Autodesk Inventor part; units mm, degrees
ref_plane "YZ Plane" through (0, 0, 0) normal (1, 0, 0) x (0, 1, 0)
ref_plane "XZ Plane" through (0, 0, 0) normal (0, 1, 0) x (-1, 0, 0)
ref_plane "XY Plane" through (0, 0, 0) normal (0, 0, 1) x (1, 0, 0)
sketch "스케치1" plane through (0, 0, 0) normal (0, 1, 0) x (-1, 0, 0)
  line L0 (0, 0) -> (-48, 0)
  line L1 (-48, 0) -> (-48, -6)
  line L2 (-48, -6) -> (0, -6)
  line L3 (0, -6) -> (0, 0)
  dimension "d0" = 48
  dimension "d1" = 6
extrude "돌출1" add sketch "스케치1" along normal blind 2
fillet "모깎기1" radius 1 7 edges at (0, 1, -6) (0, 1, 0) (0, 2, -3) (24, 2, -6) (48, 2, -3) (24, 2, 0) (48, 1, -6)
fillet "모깎기2" radius 1 2 edges at (47.7071, 1.7071, -0.2929) (48, 0.5, 0)
properties part number "gojung"
Can you work these out from the model? Positions are in its coordinate system, mm. Give positions to 0.01 mm unless a question says otherwise; leave off trailing zeros. Order: outer loops, then holes, each group sorted by start corner. A loop starts at its lowest first (then second) coordinate and runs counter-clockwise, first axis right, second up. Notation, with made-up numbers: M 84,5.5 L 127,5.5 A13 ccw 127,29.5 Z; hole C 87,53.25 d3. An arc over 180 degrees is marked long. One line per item, written item: value.
1) I want a section at A-A, the plane x = 33. List the corners of the cut face in (y, z) for me.
Answer sheet:
outline: M 0,-6 L 1,-6 A1 ccw 2,-5 L 2,-1 A1 ccw 1,0 L 0,0 Z
2) I want a section at B-B, the plane y = 1.6. List the corners of the cut face in (x, z) for me, plus the area to 3 significant figures.
Answer sheet:
outline: M 0.2,-5 A0.8 ccw 1,-5.8 L 47,-5.8 A0.8 ccw 47.8,-5 L 47.8,-1 A0.8 ccw 47,-0.2 L 1,-0.2 A0.8 ccw 0.2,-1 Z
area: 266 mm^2
3) I want a section at C-C, the plane z = -5.4. List the corners of the cut face in (x, y) for me, plus the area to 3 significant figures.
Answer sheet:
outline: M 0.08,0 L 47.92,0 L 47.92,1 A0.92 ccw 47,1.92 L 1,1.92 A0.92 ccw 0.08,1 Z
area: 91.3 mm^2
4) Please list where these lines run through material, in increasing order: line 1 along Y through (x, z) = (14, -5.1); line 2 along Z through (x, y) = (22.5, 1.1); line 3 along X through (y, z) = (1.1, -2.4).
Answer sheet:
line 1: y = 0 to 1.99
line 2: z = -5.99 to -0.01
line 3: x = 0.01 to 47.99
5) We'd pull the mould along X, two halves only. Please class faces 1 (the face through (0.285, 0.507, -0.301)), 2 (the face through (47.699, 1.715, -3.028)), 3 (the face through (24.3, 0.5, -6)): released by +X, released by -X, zero draft, split by the parting line, or undercut.
Answer sheet:
face 1: released by -X
face 2: released by +X
face 3: zero draft
